The listing builds one solid part. Answer for the finished solid, in the listing's coordinates (mm). A direction names the side the tool comes from. Round coordinates to 2 decimals unless told otherwise and drop trailing zeros. Write each loop counter-clockwise with the first axis right and the second up, starting at its lowest first coordinate (ties: lowest second). Pieces come first, ordered by that corner, then holes. Notation, with made-up numbers: (23, 44.5) -> (37, 44.5) arc R10 cw to (37, 49.5) -> close; hole circle Ø10 at (53.25, 44.5). An arc over 180 degrees is marked (long way). Write each question's results on one line, items separated by ' | '. Start each with the question number.
```python
from build123d import *

# Parameters (mm, degrees)
SKETCH1_R           = 1.6
BOSS_EXTRUDE1_DEPTH = 3
BOSS_EXTRUDE2_DEPTH = 10
SKETCH4_W           = 24
SKETCH4_H           = 30
BOSS_EXTRUDE3_DEPTH = 36
SKETCH5_W           = 14
SKETCH5_H           = 46.886122037
CUT_EXTRUDE1_DEPTH  = 10
FILLET1_R           = 10
SKETCH6_R           = 2
CUT_EXTRUDE2_DEPTH  = 17
SKETCH7_W           = 9
SKETCH7_H           = 10
CUT_EXTRUDE3_DEPTH  = 43


with BuildPart() as part:
    # Sketch1 → Boss-Extrude1 (new body)
    with BuildSketch(Plane(origin=(0, 0, 0), x_dir=(-1, 0, 0), z_dir=(0, 1, 0))):
        with BuildLine():
            Line((60, 65), (-60, 65))
            add(Edge.make_bspline(
                [(-60, 65), (-60.182819281, 65), (-60.361318877, 64.975540463), (-60.710305196, 64.881249752), (-60.880306062, 64.810741327), (-61.195311527, 64.634632862), (-61.344175944, 64.527049534), (-61.613989028, 64.285865538), (-61.735638417, 64.152370239), (-62.06437147, 63.716635859), (-62.227421468, 63.389720941), (-62.445894576, 62.69875639), (-62.5, 62.340611149), (-62.5, 61.976586008)],
                knots=[0, 0, 0, 0, 0.125, 0.125, 0.25, 0.25, 0.375, 0.375, 0.5, 0.5, 0.75, 0.75, 1, 1, 1, 1], degree=3))
            Line((-62.5, 61.976586008), (-62.5, -62.5))
            ThreePointArc((-62.5, -62.5), (-61.767766953, -64.267766953), (-60, -65))
            Line((-60, -65), (60, -65))
            ThreePointArc((60, -65), (61.767766953, -64.267766953), (62.5, -62.5))
            Line((62.5, -62.5), (62.5, 61.976586008))
            add(Edge.make_bspline(
                [(62.5, 61.976586008), (62.5, 62.34175037), (62.44618995, 62.696231112), (62.283935978, 63.211763232), (62.214956517, 63.382489596), (62.051620496, 63.705029242), (61.957290328, 63.857858356), (61.741427498, 64.145383151), (61.618346212, 64.281498062), (61.347304427, 64.524712758), (61.20089923, 64.631048566), (60.883593427, 64.80935119), (60.713329195, 64.880102966), (60.36541887, 64.974755775), (60.183838083, 65), (60, 65)],
                knots=[0, 0, 0, 0, 0.25, 0.25, 0.375, 0.375, 0.5, 0.5, 0.625, 0.625, 0.75, 0.75, 0.875, 0.875, 1, 1, 1, 1], degree=3))
        make_face()
        with Locations((60, 61.976586008)):
            Circle(SKETCH1_R, mode=Mode.SUBTRACT)
        with Locations((-60, 61.976586008)):
            Circle(SKETCH1_R, mode=Mode.SUBTRACT)
        with Locations((-60, 0.023413992)):
            Circle(SKETCH1_R, mode=Mode.SUBTRACT)
        with Locations((60, 0.023413992)):
            Circle(SKETCH1_R, mode=Mode.SUBTRACT)
        with Locations((-60, -61.976586008)):
            Circle(SKETCH1_R, mode=Mode.SUBTRACT)
        with Locations((60, -61.976586008)):
            Circle(SKETCH1_R, mode=Mode.SUBTRACT)
    extrude(amount=BOSS_EXTRUDE1_DEPTH)

    # Sketch2 → Boss-Extrude2 (add)
    with BuildSketch(Plane(origin=(0, 3, 0), x_dir=(1, 0, 0), z_dir=(0, 1, 0))):
        with BuildLine():
            Line((-62.5, -29.161742213), (62.5, -27.875786008))
            Line((62.5, -27.875786008), (62.5, -7.87481403))
            Line((62.5, -7.87481403), (56.297106888, -7.87481403))
            ThreePointArc((56.297106888, -7.87481403), (53.468679763, -6.703241155), (52.297106888, -3.87481403))
            Line((52.297106888, -3.87481403), (52.297106888, 4.677057962))
            ThreePointArc((52.297106888, 4.677057962), (53.468679763, 7.505485087), (56.297106888, 8.677057962))
            Line((56.297106888, 8.677057962), (62.5, 8.677057962))
            Line((62.5, 8.677057962), (62.5, 52.543812316))
            Line((62.5, 52.543812316), (55.701817461, 52.543812316))
            ThreePointArc((55.701817461, 52.543812316), (52.873390337, 53.715385191), (51.701817461, 56.543812316))
            Line((51.701817461, 56.543812316), (51.701817461, 65))
            Line((51.701817461, 65), (-51.729569497, 65))
            Line((-51.729569497, 65), (-51.729569497, 57.468140355))
            ThreePointArc((-51.729569497, 57.468140355), (-52.901142372, 54.63971323), (-55.729569497, 53.468140355))
            Line((-55.729569497, 53.468140355), (-62.5, 53.468140355))
            Line((-62.5, 53.468140355), (-62.5, 8.709965682))
            Line((-62.5, 8.709965682), (-55.456914608, 8.709965682))
            ThreePointArc((-55.456914608, 8.709965682), (-52.628487483, 7.538392807), (-51.456914608, 4.709965682))
            Line((-51.456914608, 4.709965682), (-51.456914608, -3.84190631))
            ThreePointArc((-51.456914608, -3.84190631), (-52.628487483, -6.670333435), (-55.456914608, -7.84190631))
            Line((-55.456914608, -7.84190631), (-62.5, -7.84190631))
            Line((-62.5, -7.84190631), (-62.5, -29.161742213))
        make_face()
        with BuildLine():
            Line((-52.5, -19.058336552), (52.5, -17.97813334))
            Line((52.5, -17.97813334), (52.5, -17.350049809))
            ThreePointArc((52.5, -17.350049809), (45.135577055, -12.325864367), (42.297106888, -3.87481403))
            Line((42.297106888, -3.87481403), (42.297106888, 4.677057962))
            ThreePointArc((42.297106888, 4.677057962), (45.135577055, 13.128108299), (52.5, 18.152293741))
            Line((52.5, 18.152293741), (52.5, 42.91485913))
            ThreePointArc((52.5, 42.91485913), (45.225378973, 47.257034801), (41.787197684, 55))
            Line((41.787197684, 55), (-41.948848065, 55))
            ThreePointArc((-41.948848065, 55), (-45.558930544, 47.847428152), (-52.5, 43.845736717))
            Line((-52.5, 43.845736717), (-52.5, 18.394141068))
            ThreePointArc((-52.5, 18.394141068), (-44.562034973, 13.502098401), (-41.456914608, 4.709965682))
            Line((-41.456914608, 4.709965682), (-41.456914608, -3.84190631))
            ThreePointArc((-41.456914608, -3.84190631), (-44.562034973, -12.634039029), (-52.5, -17.526081697))
            Line((-52.5, -17.526081697), (-52.5, -19.058336552))
        make_face(mode=Mode.SUBTRACT)
    extrude(amount=BOSS_EXTRUDE2_DEPTH)

    # Sketch4 → Boss-Extrude3 (add)
    with BuildSketch(Plane(origin=(0, 3, 0), x_dir=(1, 0, 0), z_dir=(0, 1, 0))):
        with Locations((0.057489953, -21.76285015)):
            Rectangle(SKETCH4_W, SKETCH4_H)
    extrude(amount=BOSS_EXTRUDE3_DEPTH)

    # Sketch5 → Cut-Extrude1 (cut)
    with BuildSketch(Plane(origin=(0, 39, 0), x_dir=(1, 0, 0), z_dir=(0, 1, 0))):
        with Locations((0.487990249, -20.167047514)):
            Rectangle(SKETCH5_W, SKETCH5_H)
    extrude(amount=-CUT_EXTRUDE1_DEPTH, mode=Mode.SUBTRACT)

    # Fillet1
    fillet1_edges = [part.edges().sort_by_distance(p)[0] for p in [
        (12.057489953, 3, 12.578520932),
        (-11.942510047, 3, 12.701972727),
    ]]
    fillet(fillet1_edges, radius=FILLET1_R)

    # Sketch6 → Cut-Extrude2 (cut)
    with BuildSketch(Plane(origin=(0, 29, 0), x_dir=(1, 0, 0), z_dir=(0, 1, 0))):
        with Locations((0.290601946, -16.047289156)):
            Circle(SKETCH6_R)
        with Locations((0.030645041, -32.251269585)):
            Circle(SKETCH6_R)
    extrude(amount=-CUT_EXTRUDE2_DEPTH, mode=Mode.SUBTRACT)

    # Sketch7 → Cut-Extrude3 (cut)
    with BuildSketch(Plane.XY.offset(36.76285015)):
        with Locations((0.102375744, 18.47840537)):
            Rectangle(SKETCH7_W, SKETCH7_H)
    extrude(amount=-CUT_EXTRUDE3_DEPTH, mode=Mode.SUBTRACT)


solid = part.part
```
Q1. The part is cut by section C-C, the plane z = -38.5. Write down the section's boundary in (x, y), then the cut area to 3 significant figures.
Q2. The part is cut by section D-D, the plane x = -31.5. Write down the section's boundary in (y, z).
Q3. For faces 4 (the flat face through (1, 3, -17)), 5 (the flat face through (4.602, 18, 22)), 6 (the flat face through (5, 21, 36.763)), 7 (the flat face through (-59, 8, -8.71)), determine the directions among +Z, -Z, +X, -X, +Y, -Y from which every point of the face is accessible in a straight line to the end or side of a thin tool.
Q4. Determine the mould class of faces 1 (the flat face through (1, 8, -55)), 2 (the cylindrical face through (-52.66, 7.93, -7.57)), 3 (the flat face through (59, 8, -52.544)) for opening direction X: pulls with the +X half, pulls with the -X half, needs draft (parallel to the pull), parting line crosses it, or undercut.
Q5. The part is cut by section A-A, the plane y = 19. Write down the section's boundary in (x, z).
Q6. Find the intervals of material crossed by line 1 (Z direction, x = -60, y = 2); line 2 (Y direction, x = 4, z = 7); line 3 (X direction, y = 5.5, z = -39.5), in increasing order.
Q7. The part is cut by section B-B, the plane y = 35. Write down the section's boundary in (x, z).
Q8. Each of these flat-tipped pins is pushed along its axis until it touches: pin 1 (11 mm diameter, centred on y = 31.5, z = 29, fed in from +X); pin 2 (1 mm diameter, centred on x = 8.5, z = -33, fed in from +Y); pin 3 (1.2 mm diameter, centred on x = 0, z = 16, fed in from +Y). Where does it stop, or does it pass through?
Answers follow:
1) outline: (-62.5, 0) -> (62.5, 0) -> (62.5, 13) -> (52.5, 13) -> (52.5, 3) -> (-52.5, 3) -> (-52.5, 13) -> (-62.5, 13) -> close | area: 575 mm^2
2) outline: (0, -65) -> (13, -65) -> (13, -55) -> (3, -55) -> (3, 18.84) -> (13, 18.84) -> (13, 28.84) -> (3, 28.84) -> (3, 65) -> (0, 65) -> close
3) face 4: +Y | face 5: +Z, -Z | face 6: +Z, +X, -X, +Y | face 7: -X, +Y
4) face 1: undercut | face 2: pulls with the -X half | face 3: needs draft
5) outline: (-11.94, 6.76) -> (-4.4, 6.76) -> (-4.4, 36.76) -> (-11.94, 36.76) -> close; (4.6, 6.76) -> (12.06, 6.76) -> (12.06, 36.76) -> (4.6, 36.76) -> close
6) line 1: -65 to -63.58, -60.38 to -1.58, 1.62 to 60.38, 63.58 to 65 | line 2: 0 to 13.48, 23.48 to 29 | line 3: -62.5 to -52.5, 52.5 to 62.5
7) outline: (-11.94, 6.76) -> (-6.51, 6.76) -> (-6.51, 36.76) -> (-11.94, 36.76) -> close; (7.49, 6.76) -> (12.06, 6.76) -> (12.06, 36.76) -> (7.49, 36.76) -> close
8) pin 1: x = 12.06 | pin 2: y = 3 | pin 3: y = 12
